Input: part model. Units: mm. Frame: model coordinates. A direction names the side the tool comes from. Coordinates: 2 decimals unless noted, no trailing zeros. Write each loop counter-clockwise with the first axis right and the second up, starting at its lowest first coordinate (ties: lowest second). Pieces come first, ordered by that corner, then holes. Notation, with made-up numbers: (75, 57) -> (94, 57) arc R24 ccw to (94, 70) -> close; hole circle Ø11 at (77, -12). An arc over 180 degrees is marked (long way). One line per question, with ' | ' between items. Start each with the question number.
```python
from build123d import *

# Parameters (mm, degrees)
CROQUIS1_W              = 55
CROQUIS1_H              = 55
SALIENTE_EXTRUIR1_DEPTH = 180
CROQUIS2_R              = 6
CORTAR_EXTRUIR1_DEPTH   = 30
CROQUIS3_R              = 4
CORTAR_EXTRUIR2_DEPTH   = 25
CROQUIS6_R              = 6
CORTAR_EXTRUIR5_DEPTH   = 12
CHAFL_N1_SIZE           = 2


with BuildPart() as part:
    # Croquis1 → Saliente-Extruir1 (new body)
    with BuildSketch(Plane.XY):
        Rectangle(CROQUIS1_W, CROQUIS1_H)
    extrude(amount=-SALIENTE_EXTRUIR1_DEPTH)

    # Croquis2 → Cortar-Extruir1 (cut)
    with BuildSketch(Plane.XY):
        Circle(CROQUIS2_R)
    extrude(amount=-CORTAR_EXTRUIR1_DEPTH, mode=Mode.SUBTRACT)

    # Croquis3 → Cortar-Extruir2 (cut)
    with BuildSketch(Plane(origin=(0, 0, -180), x_dir=(-1, 0, 0), z_dir=(0, 0, -1))):
        with Locations((18, 18)):
            Circle(CROQUIS3_R)
        with Locations((-18, 18)):
            Circle(CROQUIS3_R)
        with Locations((-18, -18)):
            Circle(CROQUIS3_R)
        with Locations((18, -18)):
            Circle(CROQUIS3_R)
    extrude(amount=-CORTAR_EXTRUIR2_DEPTH, mode=Mode.SUBTRACT)

    # Croquis6 → Cortar-Extruir5 (cut)
    with BuildSketch(Plane(origin=(0, 27.5, 0), x_dir=(1, 0, 0), z_dir=(0, 1, 0))):
        with Locations(Location((-18, 140, 0), (0, 0, 270))):
            Circle(CROQUIS6_R)
        with Locations(Location((18, 140, 0), (0, 0, 270))):
            Circle(CROQUIS6_R)
    extrude(amount=-CORTAR_EXTRUIR5_DEPTH, mode=Mode.SUBTRACT)

    # Chaflán1
    chafl_n1_edges = [part.edges().sort_by_distance(p)[0] for p in [
        (0, -27.5, 0),
        (-27.5, 0, 0),
        (0, 27.5, 0),
        (27.5, 0, 0),
    ]]
    chamfer(chafl_n1_edges, length=CHAFL_N1_SIZE)


solid = part.part
```
1) First-contact query: P1, Ø9.5, axis at x = 0, y = 0, coming from the +Z side; P2, Ø11, axis at x = 18, z = -140, coming from the +Y side; P3, Ø4, axis at x = 16.5, y = -18, coming from the -Z side. Flat tips, straight axial feed; report the tip coordinate or a pass-through.
2) Section C-C, the plane x = 0. Return loops of the section in (y, z).
3) Pull-direction query (Z, two-part tool) for faces 1 (the face through (-6, 0, -15)), 2 (the face through (0, 0, -30)), 3 (the face through (-21.65, 21.58, -144.76)); classes: released by +Z, released by -Z, zero draft, split by the parting line, or undercut.
4) Section A-A, the plane y = 18. Return loops of the section in (x, z), then the cut area to 3 significant figures.
5) Access query for faces 4 (the face through (-15.05, 20.7, -167.68)), 5 (the face through (18, 15.5, -140)), 6 (the face through (-27.5, 0, -90)). Directions: +Z, -Z, +X, -X, +Y, -Y. A direction counts if a zero-diameter tool reaches every point of the face in a straight line with its end or side. Return the directions, or none.
6) Section B-B, the plane z = -20.5. Return loops of the section in (x, y).
7) Ray query, line 1 (X direction, y = 20, z = -140); line 2 (Y direction, x = 18, z = -166); line 3 (Y direction, x = 0, z = -13). Return the intervals inside material, ascending.
Answer block:
1) P1: stops at z = -30 | P2: stops at y = 15.5 | P3: stops at z = -155
2) outline: (-27.5, -180) -> (27.5, -180) -> (27.5, -2) -> (25.5, 0) -> (6, 0) -> (6, -30) -> (-6, -30) -> (-6, 0) -> (-25.5, 0) -> (-27.5, -2) -> close
3) face 1: zero draft | face 2: released by +Z | face 3: undercut
4) outline: (-27.5, -180) -> (-22, -180) -> (-22, -155) -> (-14, -155) -> (-14, -180) -> (14, -180) -> (14, -155) -> (22, -155) -> (22, -180) -> (27.5, -180) -> (27.5, -2) -> (25.5, 0) -> (-25.5, 0) -> (-27.5, -2) -> close; hole circle Ø12 at (-18, -140); hole circle Ø12 at (18, -140) | area: 9,270 mm2
5) face 4: -Z | face 5: +Y | face 6: +Z, -Z, -X, +Y, -Y
6) outline: (-27.5, -27.5) -> (27.5, -27.5) -> (27.5, 27.5) -> (-27.5, 27.5) -> close; hole circle Ø12 at (0, 0)
7) line 1: x = -27.5 to -24, -12 to 12, 24 to 27.5 | line 2: y = -27.5 to -22, -14 to 14, 22 to 27.5 | line 3: y = -27.5 to -6, 6 to 27.5
